Read the model definition and answer for the solid it produces. Units are mm, in the model's axes. A direction names the side the tool comes from. Give positions to 0.01 mm unless a question says otherwise; leave off trailing zeros. Loops run counter-clockwise (first coordinate to the right, second up) from the corner with the lowest first, then second, coordinate; pieces in that order, holes last. Notation, with made-up numbers: M 4.25,45.5 L 49.25,45.5 A19 cw 49.25,51.5 Z; hole C 20,10 d1. An arc over 180 degrees is marked long. Return JSON: item names as keys, results as strings. Group by question number.
```python
from build123d import *

# Parameters (mm, degrees)
F0_R     = 1.575
F0_R_2   = 13.5
F0_W     = 4
F0_H     = 21.15
F0_W_2   = 19
F0_H_2   = 4
F1_DEPTH = 2
F2_DEPTH = 18
F4_W     = 3
F4_H     = 9.4722927755
F4_W_2   = 9
F5_DEPTH = 12
F6_R     = 1.5
F7_DEPTH = 12.5
F3_R     = 6.05
F8_DEPTH = 25
F9_R     = 1.99999
F10_SIZE = 3


# Not quite as in the source:
# - a fillet or chamfer is up to 0.001 mm smaller than in the source, because OpenCascade refuses the exact size


with BuildPart() as f1:
    # F0 (on Front) → F1 (new body)
    with BuildSketch(Plane.XZ):
        Polygon((21.15, 17.0487806691), (17.0487806691, 21.15), (-17.0487806691, 21.15), (-21.15, 17.0487806691), (-21.15, 0), (-21.15, -21.15), (-10.15, -21.15), (15.15, -21.15), (21.15, -21.15), (21.15, 0), align=None)
        with Locations((-15.5, -15.5)):
            Circle(F0_R, mode=Mode.SUBTRACT)
        with Locations((15.5, -15.5)):
            Circle(F0_R, mode=Mode.SUBTRACT)
        Circle(F0_R_2, mode=Mode.SUBTRACT)
        with Locations((-15.5, 15.5)):
            Circle(F0_R, mode=Mode.SUBTRACT)
        with Locations((15.5, 15.5)):
            Circle(F0_R, mode=Mode.SUBTRACT)
        Polygon((-21.15, -21.15), (-21.15, 0), (-25.15, 0), (-25.15, -25.15), (-10.15, -25.15), (-10.15, -21.15), align=None)
        Polygon((25.15, -21.15), (21.15, -21.15), (15.15, -21.15), (15.15, -25.15), (25.15, -25.15), align=None)
        with Locations((23.15, -10.575)):
            Rectangle(F0_W, F0_H)
        with Locations((34.65, -23.15)):
            Rectangle(F0_W_2, F0_H_2)
    extrude(amount=F1_DEPTH)

    # F0 (on Front) → F2 (join)
    with BuildSketch(Plane.XZ):
        Polygon((-21.15, -21.15), (-21.15, 0), (-25.15, 0), (-25.15, -25.15), (-10.15, -25.15), (-10.15, -21.15), align=None)
        Polygon((25.15, -21.15), (21.15, -21.15), (15.15, -21.15), (15.15, -25.15), (25.15, -25.15), align=None)
        with Locations((34.65, -23.15)):
            Rectangle(F0_W_2, F0_H_2)
        with Locations((23.15, -10.575)):
            Rectangle(F0_W, F0_H)
    extrude(amount=F2_DEPTH)

    # F4 (on face) → F5 (join)
    with BuildSketch(Plane(origin=(-25.15, 0, 0), x_dir=(0, -1, 0), z_dir=(-1, 0, 0))):
        with Locations((1.5, -20.4138536122)):
            Rectangle(F4_W, F4_H)
        with Locations((13.5, -20.4138536122)):
            Rectangle(F4_W_2, F4_H)
    extrude(amount=F5_DEPTH)

    # F6 (on face) → F7 (cut, symmetric)
    with BuildSketch(Plane.XZ.offset(3)):
        with Locations((-34.15, -20.4138536122)):
            Circle(F6_R)
    extrude(amount=F7_DEPTH, both=True, mode=Mode.SUBTRACT)

    # F3 (on face) → F8 (cut)
    with BuildSketch(Plane.XY.offset(-21.15)):
        with Locations((34.65, -9.5)):
            Circle(F3_R)
    extrude(amount=-F8_DEPTH, mode=Mode.SUBTRACT)

    # F9 (radius 2 in the source; OpenCascade refuses exactly that, so slightly less here)
    f9_edges = [f1.edges().sort_by_distance(p)[0] for p in [
        (-25.15, -1.5, -15.677707),
        (-37.15, -1.5, -15.677707),
        (-37.15, -1.5, -25.15),
        (-37.15, -13.5, -15.677707),
        (-37.15, -13.5, -25.15),
        (-25.15, -13.5, -15.677707),
        (-10.15, -9, -25.15),
        (15.15, -9, -25.15),
        (44.15, -9, -25.15),
        (44.15, -9, -21.15),
        (25.15, -9, 0),
        (21.15, -10, 0),
        (-21.15, -10, 0),
        (-25.15, -9, 0),
    ]]
    fillet(f9_edges, radius=F9_R)

    # F10
    f10_edges = [f1.edges().sort_by_distance(p)[0] for p in [
        (21.15, -10, -21.15),
        (-21.15, -10, -21.15),
    ]]
    chamfer(f10_edges, length=F10_SIZE)


solid = f1.part
```
1. For faces 4 (the cylindrical face through (-35.256, -1.521, -19.4)), 5 (the flat face through (-31, -13, -15.678)), 6 (the flat face through (0, -2, -14)), 7 (the flat face through (22, -1, 0)), determine the directions among +Z, -Z, +X, -X, +Y, -Y from which every point of the face is accessible in a straight line to the end or side of a thin tool.
2. Flat-ended cylindrical pins translate along their axes: P1, Ø21, axis at x = -1.5, z = 5, coming from the -Y side; P2, Ø6.5, axis at x = -29.5, y = -12, coming from the +Z side; P3, Ø4, axis at x = 30.5, y = -8.5, coming from the +Z side; P4, Ø8, axis at x = 15.5, y = -12.5, coming from the -Z side. Find the tip coordinate at first contact, or state that the pin passes through.
3. Find section B-B (x = 34.65). Write down the section's boundary in (y, z).
4. The mould has two halves that part along X. Classify faces 1 (the cylindrical face through (-14.045, -0.986, 14.897)), 2 (the cylindrical face through (-36.55, -13.56, -24.58)), 3 (the flat face through (-23, -9, -25.15)): +X half, -X half, draft (parallel to the pull), parting line (faces both ways), or undercut.
5. Find section A-A (x = -34.15). Write down the section's boundary in (y, z).
6. Straight lines are drawn through the part: line 1 along Z through (x, y) = (-15.5, -1.25) (3 decimals); line 2 along Z through (x, y) = (0, -1); line 3 along X through (y, z) = (-5.5, -3). For each, find the intervals that lie inside material, in ascending order.
7. Find section C-C (y = -11.75). State how many separate pieces and enclosed holes the cut face has, and give its area (3 significant figures).
8. Find section D-D (z = 1.5). Write down the section's boundary in (x, y), and give its area (3 significant figures).
Result:
{
 "1": {"face 4": "+Y", "face 5": "+Z, -X, +Y, -Y", "face 6": "+Z, -Y", "face 7": "+Z, +X, +Y, -Y"},
 "2": {"P1": "stops at y = -2", "P2": "stops at z = -15.46", "P3": "stops at z = -21.15", "P4": "stops at z = -25.15"},
 "3": {"outline": "M -18,-25.15 L -15.55,-25.15 L -15.55,-21.15 L -18,-21.15 Z; M -3.45,-25.15 L 0,-25.15 L 0,-21.15 L -3.45,-21.15 Z"},
 "4": {"face 1": "undercut", "face 2": "-X half", "face 3": "draft"},
 "5": {"outline": "M -18,-25.15 L -9,-25.15 L -9,-21.91 L -15.5,-21.91 L -15.5,-18.91 L -9,-18.91 L -9,-15.68 L -18,-15.68 Z; M -3,-25.15 L 0,-25.15 L 0,-21.91 L -3,-21.91 Z; M -3,-18.91 L 0,-18.91 L 0,-15.68 L -3,-15.68 Z"},
 "6": {"line 1": "z = -25.15 to -17.075, -13.925 to 13.925, 17.075 to 21.15", "line 2": "z = -21.15 to -13.5, 13.5 to 21.15", "line 3": "x = -25.15 to -21.15, 21.15 to 25.15"},
 "7": {"separate pieces": "3", "enclosed holes": "1", "area": "408 mm2"},
 "8": {"outline": "M -21.15,-2 L -13.42,-2 L -13.42,0 L -21.15,0 Z; M 13.42,-2 L 21.15,-2 L 21.15,0 L 13.42,0 Z", "area": "30.9 mm2"}
}
